The listing builds one solid part. Answer for the finished solid, in the listing's coordinates (mm). Face numbers are marked on the shaded views. A direction names the side the tool comes from. Give positions to 0.01 mm unless a question says otherwise; leave off trailing zeros. Loops run counter-clockwise (first coordinate to the right, second up) from the corner with the lowest first, then second, coordinate; pieces in that order, holes last. Notation, with made-up numbers: M 22,56.5 L 27,56.5 A34 ccw 27,92.5 Z; hole C 0.25,66 d10. An arc over 180 degrees is marked long. Use one line per item in the form item = value. Start each with the question number.
1. The mould has two halves that part along X. Classify the marked faces 3, 4, 5 and 6: released by +X, released by -X, zero draft, split by the parting line, or undercut.
2. The part is cut by section A-A (y = 1.3). Give the number of separate pieces and of enclosed holes in the cut face, and give its area (3 significant figures).
3. Straight lines are drawn through the part: line 1 (X direction, y = 1.75, z = -7) (3 decimals); line 2 (X direction, y = 1.25, z = -8.5) (3 decimals); line 3 (Z direction, x = 3.75, y = 1.75) (3 decimals). For each, find the intervals that lie inside material, in ascending order. Write a range as from..to.
4. The part is cut by section D-D (x = 6.5). Write down the section's boundary in (y, z) (3 decimals).
5. The part is cut by section B-B (x = 1.25). Write down the section's boundary in (y, z) (3 decimals).
6. The part is cut by section C-C (z = -2). Write down the section's boundary in (x, y) (3 decimals), and give its area (3 significant figures).
7. For the marked faces 1 and 2, determine the directions among +Z, -Z, +X, -X, +Y, -Y from which every point of the face is accessible in a straight line to the end or side of a thin tool.
8. This flat-tipped pin is pushed along its axis until it touches: pin 1 Ø1 at (x, z) = (4, -6) entering from +Y. Where does it stop, or does it pass through?
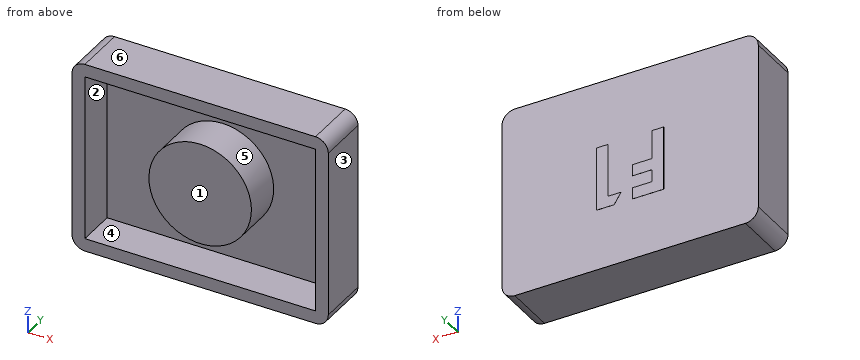
from build123d import *

# Parameters (mm, degrees)
SKETCH1_W           = 12.7
SKETCH1_H           = 9.525
BOSS_EXTRUDE1_DEPTH = 2.54
FILLET1_R           = 0.635
SHELL1_START        = 0.635
SHELL1_OUTLINE_W    = 1.905
SHELL1_OUTLINE_H    = 8.255
SHELL1_DEPTH        = 11.43
SKETCH2_R           = 2.54
BOSS_EXTRUDE2_DEPTH = 1.905
BOSS_EXTRUDE3_DEPTH = 0.00254


# Read off the part's stored shape, not the designer's step: Shell1
with BuildPart() as part:
    # Sketch1 → Boss-Extrude1 (new body)
    with BuildSketch(Plane(origin=(0, 0, 0), x_dir=(1, 0, 0), z_dir=(0, 1, 0))):
        with Locations((6.35, 4.7625)):
            Rectangle(SKETCH1_W, SKETCH1_H)
    extrude(amount=BOSS_EXTRUDE1_DEPTH)

    # Fillet1
    fillet1_edges = [part.edges().sort_by_distance(p)[0] for p in [
        (0, 1.27, -9.525),
        (12.7, 1.27, -9.525),
        (12.7, 1.27, 0),
        (0, 1.27, 0),
    ]]
    fillet(fillet1_edges, radius=FILLET1_R)

    # Shell1 outline → Shell1 (cut)
    with BuildSketch(Plane.YZ.offset(SHELL1_START)):
        with Locations((0.9525, -4.7625)):
            Rectangle(SHELL1_OUTLINE_W, SHELL1_OUTLINE_H)
    extrude(amount=SHELL1_DEPTH, mode=Mode.SUBTRACT)

    # Sketch2 → Boss-Extrude2 (add)
    with BuildSketch(Plane(origin=(0, 1.905, 0), x_dir=(-1, 0, 0), z_dir=(0, -1, 0))):
        with Locations(Location((-6.35, 4.7625, 0), (0, 0, 270))):
            Circle(SKETCH2_R)
    extrude(amount=BOSS_EXTRUDE2_DEPTH)

    # Sketch3 → Boss-Extrude3 (add)
    with BuildSketch(Plane(origin=(0, 2.54, 0), x_dir=(1, 0, 0), z_dir=(0, 1, 0))):
        Polygon((4.684346154, 6.477), (6.231141026, 6.477), (6.231141026, 5.907128205), (5.254217949, 5.907128205), (5.254217949, 5.296551282), (6.231141026, 5.296551282), (6.231141026, 4.726679487), (5.254217949, 4.726679487), (5.254217949, 3.302), (4.684346154, 3.302), align=None)
        Polygon((7.141282252, 6.477), (8.022166667, 6.477), (8.022166667, 3.302), (7.452294872, 3.302), (7.452294872, 5.947833333), (6.801012821, 5.947833333), align=None)
    extrude(amount=BOSS_EXTRUDE3_DEPTH)


solid = part.part
Derived:
q1.face_3 = released by +X
q1.face_4 = undercut
q1.face_5 = undercut
q1.face_6 = zero draft
q2.separate_pieces = 2
q2.enclosed_holes = 1
q2.area = 46.5 mm2
q3.line_1 = 0..0.635, 5.148..7.552, 12.065..12.7
q3.line_2 = 0..0.635, 12.065..12.7
q3.line_3 = -9.525..-8.89, -0.635..0
q4.outline = M 0,-9.525 L 2.54,-9.525 L 2.54,0 L 0,0 L 0,-0.635 L 1.905,-0.635 L 1.905,-2.227 L 0,-2.227 L 0,-7.298 L 1.905,-7.298 L 1.905,-8.89 L 0,-8.89 Z
q5.outline = M 0,-9.525 L 2.54,-9.525 L 2.54,0 L 0,0 L 0,-0.635 L 1.905,-0.635 L 1.905,-8.89 L 0,-8.89 Z
q6.outline = M 0,0 L 0.635,0 L 0.635,1.905 L 12.065,1.905 L 12.065,0 L 12.7,0 L 12.7,2.54 L 0,2.54 Z
q6.area = 10.5 mm2
q7.face_1 = +Z, -Z, +X, -X, -Y
q7.face_2 = -Y
q8.pin_1 = 2.54
